from build123d import *

# Parameters (mm, degrees)
SKETCH1_W           = 145
SKETCH1_H           = 45
BOSS_EXTRUDE1_DEPTH = 5
CUT_EXTRUDE1_DEPTH  = 77.075620274
FILLET1_R           = 5
FILLET2_R           = 5
FILLET3_R           = 5
FILLET4_R           = 5
SKETCH3_R           = 2.5
CUT_EXTRUDE2_DEPTH  = 77.075620274
SKETCH4_R           = 15
CUT_EXTRUDE3_DEPTH  = 77.075620274


with BuildPart() as part:
    # Sketch1 → Boss-Extrude1 (new body)
    with BuildSketch(Plane(origin=(0, 0, 0), x_dir=(1, 0, 0), z_dir=(0, 1, 0))):
        Rectangle(SKETCH1_W, SKETCH1_H)
    extrude(amount=BOSS_EXTRUDE1_DEPTH)

    # Sketch2 → Cut-Extrude1 (cut, through all)
    with BuildSketch(Plane(origin=(0, 5, 0), x_dir=(1, 0, 0), z_dir=(0, 1, 0))):
        with BuildLine():
            Line((-67.5, 8.35), (-47.5, 8.35))
            ThreePointArc((-47.5, 8.35), (-45.85, 10), (-47.5, 11.65))
            Line((-47.5, 11.65), (-67.5, 11.65))
            ThreePointArc((-67.5, 11.65), (-69.15, 10), (-67.5, 8.35))
        make_face()
        with BuildLine():
            Line((-47.5, -11.65), (-67.5, -11.65))
            ThreePointArc((-67.5, -11.65), (-69.15, -10), (-67.5, -8.35))
            Line((-67.5, -8.35), (-47.5, -8.35))
            ThreePointArc((-47.5, -8.35), (-45.85, -10), (-47.5, -11.65))
        make_face()
        with BuildLine():
            Line((47.5, 11.65), (67.5, 11.65))
            ThreePointArc((67.5, 11.65), (69.15, 10), (67.5, 8.35))
            Line((67.5, 8.35), (47.5, 8.35))
            ThreePointArc((47.5, 8.35), (45.85, 10), (47.5, 11.65))
        make_face()
        with BuildLine():
            Line((47.5, -11.65), (67.5, -11.65))
            ThreePointArc((67.5, -11.65), (69.15, -10), (67.5, -8.35))
            Line((67.5, -8.35), (47.5, -8.35))
            ThreePointArc((47.5, -8.35), (45.85, -10), (47.5, -11.65))
        make_face()
    extrude(amount=-CUT_EXTRUDE1_DEPTH, mode=Mode.SUBTRACT)

    # Fillet1
    fillet1_edges = [part.edges().sort_by_distance(p)[0] for p in [
        (72.5, 2.5, -22.5),
    ]]
    fillet(fillet1_edges, radius=FILLET1_R)

    # Fillet2
    fillet2_edges = [part.edges().sort_by_distance(p)[0] for p in [
        (-72.5, 2.5, -22.5),
    ]]
    fillet(fillet2_edges, radius=FILLET2_R)

    # Fillet3
    fillet3_edges = [part.edges().sort_by_distance(p)[0] for p in [
        (-72.5, 2.5, 22.5),
    ]]
    fillet(fillet3_edges, radius=FILLET3_R)

    # Fillet4
    fillet4_edges = [part.edges().sort_by_distance(p)[0] for p in [
        (72.5, 2.5, 22.5),
    ]]
    fillet(fillet4_edges, radius=FILLET4_R)

    # Sketch3 → Cut-Extrude2 (cut, through all)
    with BuildSketch(Plane(origin=(0, 5, 0), x_dir=(1, 0, 0), z_dir=(0, 1, 0))):
        with Locations(Location((30.310889132, 17.5, 0), (0, 0, 270))):
            Circle(SKETCH3_R)
        with Locations(Location((30.310889132, -17.5, 0), (0, 0, 270))):
            Circle(SKETCH3_R)
        with Locations(Location((-30.310889132, -17.5, 0), (0, 0, 270))):
            Circle(SKETCH3_R)
        with Locations(Location((-30.310889132, 17.5, 0), (0, 0, 270))):
            Circle(SKETCH3_R)
    extrude(amount=-CUT_EXTRUDE2_DEPTH, mode=Mode.SUBTRACT)

    # Sketch4 → Cut-Extrude3 (cut, through all)
    with BuildSketch(Plane(origin=(0, 5, 0), x_dir=(1, 0, 0), z_dir=(0, 1, 0))):
        with Locations(Location((0, 0, 0), (0, 0, 270))):
            Circle(SKETCH4_R)
    extrude(amount=-CUT_EXTRUDE3_DEPTH, mode=Mode.SUBTRACT)


solid = part.part
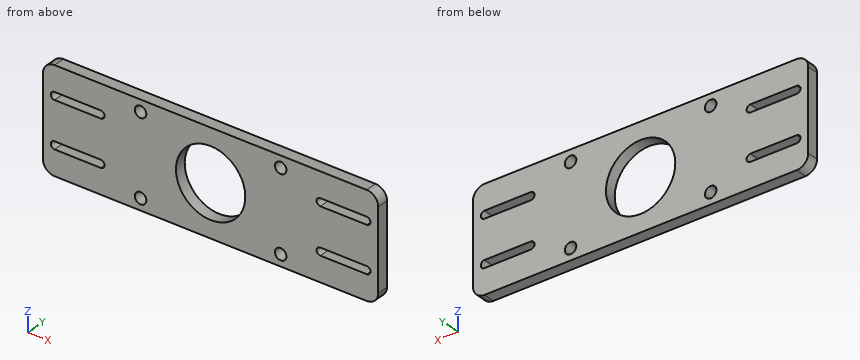
Work out the finished part from the listing and answer in its coordinate system (mm). Coordinates: 2 decimals unless noted, no trailing zeros. Write each loop counter-clockwise with the first axis right and the second up, starting at its lowest first coordinate (ties: lowest second). Pieces come first, ordered by that corner, then holes. Notation, with made-up numbers: M 43,66 L 73,66 A13 ccw 73,80 Z; hole C 77,80 d9. An arc over 180 degrees is marked long. Write item = value, one per line.
1. The part is cut by section A-A (x = 0). Determine the outline of the cut face in (y, z).
Solution:
outline = M 0,-22.5 L 5,-22.5 L 5,-15 L 0,-15 Z; M 0,15 L 5,15 L 5,22.5 L 0,22.5 Z
2. The part is cut by section C-C (z = 0). Determine the outline of the cut face in (x, y).
Solution:
outline = M -72.5,0 L -15,0 L -15,5 L -72.5,5 Z; M 15,0 L 72.5,0 L 72.5,5 L 15,5 Z
3. The part is cut by section D-D (z = 10). Determine the outline of the cut face in (x, y), then the cut area to 3 significant figures.
Solution:
outline = M -72.5,0 L -69.15,0 L -69.15,5 L -72.5,5 Z; M -45.85,0 L -11.18,0 L -11.18,5 L -45.85,5 Z; M 11.18,0 L 45.85,0 L 45.85,5 L 11.18,5 Z; M 69.15,0 L 72.5,0 L 72.5,5 L 69.15,5 Z
area = 380 mm2
4. Straight lines are drawn through the part: line 1 (Z direction, x = 60, y = 3.7); line 2 (X direction, y = 1.15, z = 17.5). For each, find the intervals that lie inside material, in ascending order. Write a range as from..to.
Solution:
line_1 = -22.5..-11.65, -8.35..8.35, 11.65..22.5
line_2 = -72.5..-32.81, -27.81..27.81, 32.81..72.5
5. The part is cut by section B-B (x = -51.5). Determine the outline of the cut face in (y, z).
Solution:
outline = M 0,-22.5 L 5,-22.5 L 5,-11.65 L 0,-11.65 Z; M 0,-8.35 L 5,-8.35 L 5,8.35 L 0,8.35 Z; M 0,11.65 L 5,11.65 L 5,22.5 L 0,22.5 Z
6. A flat-ended cylindrical pin translates along its axis: pin 1 (4.5 mm diameter, centred on x = 30.31, z = 17.5, fed in from +Y). Find the tip coordinate at first contact, or state that the pin passes through.
Solution:
pin_1 = through
